Model file for the job. Use its own axes, mm. A direction names the side the tool comes from. Round coordinates to 2 decimals unless told otherwise and drop trailing zeros. Write each loop counter-clockwise with the first axis right and the second up, starting at its lowest first coordinate (ties: lowest second). Pieces come first, ordered by that corner, then holes.
```python
from build123d import *

# Parameters (mm, degrees)
F0_W     = 500
F0_H     = 800
F1_DEPTH = 1000
F2_R     = 125
F3_DEPTH = 25
F4_R     = 249.99999
F6_DEPTH = 25
F7_W     = 600
F7_H     = 8.0311238766
F8_DEPTH = 100


# Not quite as in the source:
# - a fillet or chamfer is up to 0.001 mm smaller than in the source, because OpenCascade refuses the exact size


with BuildPart() as f1:
    # F0 (on Right) → F1 (new body)
    with BuildSketch(Plane.YZ):
        Rectangle(F0_W, F0_H)
    extrude(amount=F1_DEPTH)

    # F2 (on face) → F3 (cut)
    with BuildSketch(Plane.YZ.offset(1000)):
        with Locations((0, 234.9280565977)):
            Circle(F2_R)
    extrude(amount=-F3_DEPTH, mode=Mode.SUBTRACT)

    # F4 (radius 250 in the source; OpenCascade refuses exactly that, so slightly less here)
    f4_edges = [f1.edges().sort_by_distance(p)[0] for p in [
        (500, 250, 400),
        (500, -250, 400),
    ]]
    fillet(f4_edges, radius=F4_R)

    # F5 (on face) → F6 (cut)
    with BuildSketch(Plane(origin=(0, 250, 0), x_dir=(-1, 0, 0), z_dir=(0, 1, 0))):
        Polygon((-300, 150), (-700, 150), (-700, -14.3443720028), (-700, -150), (-300, -150), align=None)
    extrude(amount=-F6_DEPTH, mode=Mode.SUBTRACT)

    # F7 (on face) → F8 (cut)
    with BuildSketch(Plane(origin=(0, 250, 0), x_dir=(-1, 0, 0), z_dir=(0, 1, 0))):
        with Locations((-500, -404.0155619383)):
            Rectangle(F7_W, F7_H)
    extrude(amount=-F8_DEPTH, mode=Mode.SUBTRACT)


solid = f1.part
```
1) Wall check: probe 1 along X at (y, z) = (-60.5, 132.5); probe 2 along Z at (x, y) = (355, 3); probe 3 along Y at (x, z) = (316.5, -110). Give the ranges that are in metal, low to high.
2) Which spindle directions (+Z, -Z, +X, -X, +Y, -Y) get a long thin tool onto all of the face, cutting with end or side? Do faces 1 (the face through (700, 238, 2)), 2 (the face through (493, -250, -129)), 3 (the face through (975, -2, 237)). Say none if no direction does.
3) Cut at C-C on y = 97. List the corners of the cut face in (x, z), and give its area (3 significant figures).
4) Pull direction Z, two halves, no side cores. Call faces 4 (the face through (507, 174.82, 328.71)), 5 (the face through (1000, -3, -83)), 6 (the face through (300, 238, -2)): released by +Z, released by -Z, zero draft, split by the parting line, or undercut.
5) Flat gauge pin, fed straight in: pin 1 Ø1.5 at (y, z) = (-72, 153.5) entering from +X. Where does the tip first touch, or does it go through?
6) Cut at A-A on z = -41. List the corners of the cut face in (x, y).
Result sheet:
1. probe 1: x = 0 to 975
1. probe 2: z = -400 to 399.98
1. probe 3: y = -250 to 225
2. face 1: +Y
2. face 2: +Z, -Z, +X, -X, -Y
2. face 3: +X
3. outline: (0, -400) - (1000, -400) - (1000, 156.09) - (975, 156.09) - (975, 313.77) - (1000, 313.77) - (1000, 380.41) - (0, 380.41) - close
3. area: 776,000 mm2
4. face 4: released by +Z
4. face 5: zero draft
4. face 6: undercut
5. pin 1: stops at x = 975
6. outline: (0, -250) - (1000, -250) - (1000, 250) - (700, 250) - (700, 225) - (300, 225) - (300, 250) - (0, 250) - close
